Geometry check sheet. Reference: the model listing, model coordinates, mm. Coordinates: 2 decimals unless noted, no trailing zeros. Write each loop counter-clockwise with the first axis right and the second up, starting at its lowest first coordinate (ties: lowest second). Pieces come first, ordered by that corner, then holes. Notation, with made-up numbers: (7, 54.5) -> (44, 54.5) arc R24 ccw to (44, 72.5) -> close; hole circle Ø1 at (23.5, 48.5). An arc over 180 degrees is marked (long way). Answer in a Markdown table with one row per item. Add a question column.
1. Scan lines: L1, parallel to Z at x = 30, y = -17.5; L2, parallel to Z at x = 31.5, y = -2.5. Record each from-to range of solid material in increasing order. Write a range as from..to.
2. Cross-section at C-C on y = -6. Give the number of separate pieces and of enclosed holes in the cut face, and give its area (3 significant figures).
3. Depth check by flat-ended pin: P1, Ø4, axis at x = 90.29, z = 60.32, coming from the -Y side. Enter the tip coordinate at first touch or a pass-through.
4. Cross-section at B-B on x = 22.5. Record the cut outline in (y, z).
5. Cross-section at A-A on z = 38.1. Record the cut outline in (x, y).
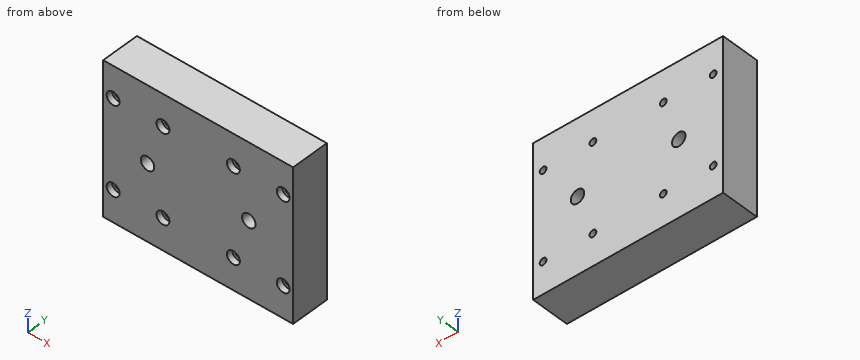
```python
from build123d import *

# Parameters (mm, degrees)
F0_W           = 95.25
F0_H           = 76.2
F1_DEPTH       = 19.05
F3_D           = 3.4
F3_CBORE_D     = 6.5
F3_CBORE_DEPTH = 3
F5_D           = 6.7564


with BuildPart() as f1:
    # F0 (on Front) → F1 (new body)
    with BuildSketch(Plane.XZ):
        with Locations((47.625, 38.1)):
            Rectangle(F0_W, F0_H)
    extrude(amount=F1_DEPTH)

    # F3 (through all)
    with Locations(Plane.XZ.offset(19.05)):
        with Locations((4.9625, 60.325), (29.9625, 60.325), (65.2875, 60.325), (90.2875, 60.325), (4.9625, 15.875), (29.9625, 15.875), (65.2875, 15.875), (90.2875, 15.875)):
            CounterBoreHole(F3_D / 2, F3_CBORE_D / 2, F3_CBORE_DEPTH)

    # F5 (through all)
    with Locations(Plane(origin=(0, 0, 0), x_dir=(-1, 0, 0), z_dir=(0, 1, 0))):
        with Locations((-73.025, 38.1), (-22.225, 38.1)):
            Hole(F5_D / 2)


solid = f1.part
```
Results found:
| question | item | result |
|---|---|---|
| 1 | L1 | z = 0..12.63, 19.12..57.08, 63.57..76.2 |
| 1 | L2 | z = 0..15.15, 16.6..59.6, 61.05..76.2 |
| 2 | separate pieces | 1 |
| 2 | enclosed holes | 10 |
| 2 | area | 7,110 mm^2 |
| 3 | P1 | stops at y = -16.05 |
| 4 | outline | (-19.05, 0) -> (0, 0) -> (0, 34.73) -> (-19.05, 34.73) -> close; (-19.05, 41.47) -> (0, 41.47) -> (0, 76.2) -> (-19.05, 76.2) -> close |
| 5 | outline | (0, -19.05) -> (18.85, -19.05) -> (18.85, 0) -> (0, 0) -> close; (25.6, -19.05) -> (69.65, -19.05) -> (69.65, 0) -> (25.6, 0) -> close; (76.4, -19.05) -> (95.25, -19.05) -> (95.25, 0) -> (76.4, 0) -> close |
